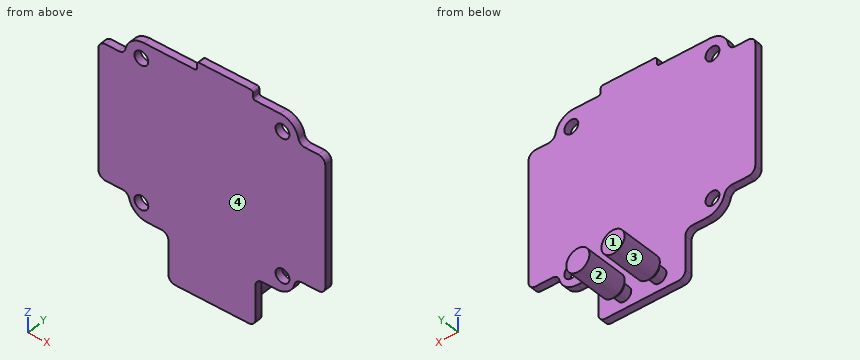
```python
from build123d import *

# Parameters (mm, degrees)
SKETCH1_R           = 1.5
BOSS_EXTRUDE1_DEPTH = 1.6
FILLET1_R           = 4
FILLET2_R           = 1.5
FILLET3_R           = 0.5
SKETCH2_R           = 1.25
BOSS_EXTRUDE2_DEPTH = 1.5
SKETCH3_R           = 1.5
BOSS_EXTRUDE3_DEPTH = 2
SKETCH4_R           = 2.5
BOSS_EXTRUDE4_DEPTH = 10
CHAMFER1_SIZE       = 0.9


with BuildPart() as part:
    # Sketch1 → Boss-Extrude1 (new body)
    with BuildSketch(Plane(origin=(0, 0, 0), x_dir=(1, 0, 0), z_dir=(0, 1, 0))):
        Polygon((3.682892501, 9.884360961), (9.432892501, 9.884360961), (9.432892501, 5.424302162), (24.937092609, 5.424302162), (24.937092609, 3.570771232), (37.100889333, 3.570771232), (37.100889333, 5.424302162), (46.932892501, 5.424302162), (46.932892501, 9.884360961), (52.682892501, 9.884360961), (52.682892501, 38.695125613), (46.161283606, 38.695125613), (46.161283606, 42.924302162), (37.585453381, 42.924302162), (37.585453381, 53.114107514), (18.780331621, 53.114107514), (18.780331621, 42.924302162), (10.204501396, 42.924302162), (10.204501396, 38.695125613), (3.682892501, 38.695125613), align=None)
        with Locations(Location((12.932892501, 8.924302162, 0), (0, 0, 270))):
            Circle(SKETCH1_R, mode=Mode.SUBTRACT)
        with Locations(Location((43.432892501, 8.924302162, 0), (0, 0, 270))):
            Circle(SKETCH1_R, mode=Mode.SUBTRACT)
        with Locations(Location((43.432892501, 39.424302162, 0), (0, 0, 270))):
            Circle(SKETCH1_R, mode=Mode.SUBTRACT)
        with Locations(Location((12.932892501, 39.424302162, 0), (0, 0, 270))):
            Circle(SKETCH1_R, mode=Mode.SUBTRACT)
    extrude(amount=BOSS_EXTRUDE1_DEPTH)

    # Fillet1
    fillet1_edges = [part.edges().sort_by_distance(p)[0] for p in [
        (46.161283606, 0.8, -42.924302162),
        (46.932892501, 0.8, -5.424302162),
        (9.432892501, 0.8, -5.424302162),
        (10.204501396, 0.8, -42.924302162),
    ]]
    fillet(fillet1_edges, radius=FILLET1_R)

    # Fillet2
    fillet2_edges = [part.edges().sort_by_distance(p)[0] for p in [
        (52.682892501, 0.8, -9.884360961),
        (52.682892501, 0.8, -38.695125613),
        (37.585453381, 0.8, -42.924302162),
        (37.585453381, 0.8, -53.114107514),
        (18.780331621, 0.8, -53.114107514),
        (18.780331621, 0.8, -42.924302162),
        (3.682892501, 0.8, -38.695125613),
        (46.932892501, 0.8, -9.884360961),
        (9.432892501, 0.8, -9.884360961),
        (46.161283606, 0.8, -38.695125613),
        (10.204501396, 0.8, -38.695125613),
        (3.682892501, 0.8, -9.884360961),
    ]]
    fillet(fillet2_edges, radius=FILLET2_R)

    # Fillet3
    fillet3_edges = [part.edges().sort_by_distance(p)[0] for p in [
        (37.100889333, 0.8, -5.424302162),
        (37.100889333, 0.8, -3.570771232),
        (24.937092609, 0.8, -3.570771232),
        (24.937092609, 0.8, -5.424302162),
    ]]
    fillet(fillet3_edges, radius=FILLET3_R)

    # Sketch2 → Boss-Extrude2 (add)
    with BuildSketch(Plane(origin=(0, 1.6, 0), x_dir=(1, 0, 0), z_dir=(0, 1, 0))):
        with Locations(Location((31.982892501, 50.114107514, 0), (0, 0, 270))):
            Circle(SKETCH2_R)
        with Locations(Location((24.382892501, 50.114107514, 0), (0, 0, 90))):
            Circle(SKETCH2_R)
    extrude(amount=BOSS_EXTRUDE2_DEPTH)

    # Sketch3 → Boss-Extrude3 (add)
    with BuildSketch(Plane(origin=(0, 1.6, 0), x_dir=(1, 0, 0), z_dir=(0, 1, 0))):
        with Locations(Location((31.982892501, 50.114107514, 0), (0, 0, 270))):
            Circle(SKETCH3_R)
        with Locations(Location((24.382892501, 50.114107514, 0), (0, 0, 270))):
            Circle(SKETCH3_R)
    extrude(amount=BOSS_EXTRUDE3_DEPTH)

    # Sketch4 → Boss-Extrude4 (add)
    with BuildSketch(Plane(origin=(0, 3.6, 0), x_dir=(1, 0, 0), z_dir=(0, 1, 0))):
        with Locations(Location((31.982892501, 50.114107514, 0), (0, 0, 270))):
            Circle(SKETCH4_R)
        with Locations(Location((24.382892501, 50.114107514, 0), (0, 0, 270))):
            Circle(SKETCH4_R)
    extrude(amount=BOSS_EXTRUDE4_DEPTH)

    # Chamfer1
    chamfer1_edges = [part.edges().sort_by_distance(p)[0] for p in [
        (31.982892501, 3.6, -52.614107514),
        (24.382892501, 3.6, -52.614107514),
    ]]
    chamfer(chamfer1_edges, length=CHAMFER1_SIZE)


solid = part.part
```
Check sheet for the modelled part. Datum: model origin and axes. Units: mm. Face numbers are marked on the shaded views. A direction names the side the tool comes from. Round coordinates to 2 decimals unless told otherwise and drop trailing zeros. Order: outer loops, then holes, each group sorted by start corner. A loop starts at its lowest first (then second) coordinate and runs counter-clockwise, first axis right, second up.
1) Section check C-C (y = 5.5). Record the boundary of the cut face in (x, z).
2) Mould release check, pull along X, two halves, no side actions. Record for the marked faces 3 and 4: +X half, -X half, draft (parallel to the pull), parting line (faces both ways), or undercut.
3) Section check B-B (x = 41). Record the boundary of the cut face in (y, z).
4) Go/stop test with flat-tipped pins: pin 1 Ø1.3 at (x, y) = (41, 0.5) entering from -Z; pin 2 Ø1.3 at (x, y) = (6.5, 0.5) entering from +Z; pin 3 Ø5 at (x, y) = (31, 5) entering from +Z; pin 4 Ø2.5 at (x, z) = (12.93, -39.42) entering from +Y. Record where each tip stops, or that it passes through.
5) Tool access check on the marked faces 1 and 2. Record the directions out of +Z, -Z, +X, -X, +Y, -Y that give a thin tool (end or side, any length) a straight path to the whole face; none if there is none.
6) Section check A-A (z = -46). Record the boundary of the cut face in (x, y).
7) Scan lines: line 1 (Y direction, x = 50.5, z = -29); line 2 (X direction, y = 5.25, z = -48); line 3 (Z direction, x = 32.5, y = 3.5). Record each from-to range of solid material in increasing order.
Result:
1. outline: circle Ø5 at (24.38, -50.11); circle Ø5 at (31.98, -50.11)
2. face 3: undercut
2. face 4: draft
3. outline: (0, -42.92) - (1.6, -42.92) - (1.6, -5.42) - (0, -5.42) - close
4. pin 1: stops at z = -42.92
4. pin 2: stops at z = -9.88
4. pin 3: stops at z = -47.61
4. pin 4: passes through
5. face 1: +Z, -Z, +X, -X, +Y
5. face 2: +Y
6. outline: (18.78, 0) - (37.59, 0) - (37.59, 1.6) - (18.78, 1.6) - close
7. line 1: y = 0 to 1.6
7. line 2: x = 23.05 to 25.72, 30.65 to 33.32
7. line 3: z = -51.52 to -48.71
